Can you work these out from the model? Positions are in its coordinate system, mm. A direction names the side the tool comes from. Give positions to 0.01 mm unless a question says otherwise; leave off trailing zeros. Loops run counter-clockwise (first coordinate to the right, second up) from the corner with the lowest first, then second, coordinate; pieces in that order, holes last. Notation, with made-up numbers: (67, 69) -> (115, 69) arc R10 ccw to (115, 75) -> close; hole circle Ø11 at (7.5, -20.75). An arc over 180 degrees is marked (long way). One line per question, with ' | ' between items.
from build123d import *

# Parameters (mm, degrees)
F0_R      = 0.6477
F0_R_2    = 0.6441405576
F1_DEPTH  = 25.4
F2_W      = 127.2426065671
F2_H      = 43.082173756
F3_DEPTH  = 25.4
F6_DEPTH  = 127.2436065671
F7_W      = 127.2426065671
F7_H      = 36.2138515522
F8_DEPTH  = 25.4
F11_DEPTH = 127.2436065671
F12_W     = 127.2426065671
F12_H     = 79.2960253082
F13_DEPTH = 2.54


# Not quite as in the source:
# - ends of sketch curves that miss each other by under 0.0002 mm in the source are joined


with BuildPart() as f1:
    # F0 (on Top) → F1 (new body)
    with BuildSketch(Plane.XY):
        Polygon((-47.2229928794, 27.8801387091), (-47.2229928794, 30.4201387091), (-44.6829928794, 30.4201387091), (2.3896338216, 30.4201387091), (2.3896338216, 33.6738515522), (2.3896338216, 36.2138515522), (-62.2987892685, 36.2138515522), (-62.2987892685, 19.4619052569), (-59.7587892685, 19.4619052569), (-47.2229928794, 19.4619052569), align=None)
        Polygon((-44.6829928794, 30.4201387091), (-47.2229928794, 30.4201387091), (-47.2229928794, 27.8801387091), (-47.2229928794, 19.4619052569), (-59.7587892685, 19.4619052569), (-62.2987892685, 19.4619052569), (-62.2987892685, 16.9219052569), (-62.2987892685, -29.6174437481), (-62.2987892685, -32.1574437481), (-59.7587892685, -32.1574437481), (-16.2234111885, -32.1574437481), (-13.6834111885, -32.1574437481), (-13.6834111885, -29.6174437481), (-13.6834111885, -19.4574437481), (9.1386072609, -19.4574437481), (9.1386072609, -40.542173756), (9.1386072609, -43.082173756), (11.6786072609, -43.082173756), (32.1430532363, -43.082173756), (34.6830532363, -43.082173756), (34.6830532363, -40.542173756), (34.6830532363, -19.4574437481), (62.4038172987, -19.4574437481), (62.4038172987, -16.9174437481), (34.6830532363, -16.9174437481), (32.1430532363, -16.9174437481), (32.1430532363, -19.4574437481), (32.1430532363, -40.542173756), (11.6786072609, -40.542173756), (11.6786072609, -19.4574437481), (11.6786072609, -16.9174437481), (9.1386072609, -16.9174437481), (-13.6834111885, -16.9174437481), (-16.2234111885, -16.9174437481), (-16.2234111885, -19.4574437481), (-16.2234111885, -29.6174437481), (-59.7587892685, -29.6174437481), (-59.7587892685, 1.3920115222), (-59.7587892685, 2.6620115222), (-59.7587892685, 16.9219052569), (-47.2229928794, 16.9219052569), (-45.9529928794, 16.9219052569), (-44.6829928794, 16.9219052569), (-44.6829928794, 19.4619052569), (-44.6829928794, 27.8801387091), (2.3896338216, 27.8801387091), (4.9296338216, 27.8801387091), (4.9296338216, 30.4201387091), (4.9296338216, 33.6738515522), (11.6786072609, 33.6738515522), (11.6786072609, 30.4201387091), (11.6786072609, 27.8801387091), (14.2186072609, 27.8801387091), (62.4038172987, 27.8801387091), (62.4038172987, 30.4201387091), (14.2186072609, 30.4201387091), (14.2186072609, 33.6738515522), (14.2186072609, 36.2138515522), (11.6786072609, 36.2138515522), (4.9296338216, 36.2138515522), (2.3896338216, 36.2138515522), (2.3896338216, 33.6738515522), (2.3896338216, 30.4201387091), align=None)
        with Locations((-61.0287892685, -30.8874437481)):
            Circle(F0_R, mode=Mode.SUBTRACT)
        with Locations((-14.9534111885, -30.8874437481)):
            Circle(F0_R, mode=Mode.SUBTRACT)
        with Locations((-14.9534111885, -18.1874437481)):
            Circle(F0_R, mode=Mode.SUBTRACT)
        with Locations((10.4086072609, -41.812173756)):
            Circle(F0_R, mode=Mode.SUBTRACT)
        with Locations((33.4130532363, -41.812173756)):
            Circle(F0_R, mode=Mode.SUBTRACT)
        with Locations((10.4086072609, -18.1874437481)):
            Circle(F0_R, mode=Mode.SUBTRACT)
        with Locations((33.4130532363, -18.1874437481)):
            Circle(F0_R, mode=Mode.SUBTRACT)
        with Locations((-61.0287892685, 18.1919052569)):
            Circle(F0_R, mode=Mode.SUBTRACT)
        with Locations((-45.9529928794, 18.1919052569)):
            Circle(F0_R, mode=Mode.SUBTRACT)
        with Locations((-45.9529928794, 29.1501387091)):
            Circle(F0_R_2, mode=Mode.SUBTRACT)
        with Locations((3.6596338216, 29.1501387091)):
            Circle(F0_R, mode=Mode.SUBTRACT)
        with Locations((12.9486072609, 29.1501387091)):
            Circle(F0_R, mode=Mode.SUBTRACT)
        with Locations((3.6596338216, 34.9438515522)):
            Circle(F0_R, mode=Mode.SUBTRACT)
        with Locations((12.9486072609, 34.9438515522)):
            Circle(F0_R, mode=Mode.SUBTRACT)
        Polygon((64.9438172987, 36.2138515522), (14.2186072609, 36.2138515522), (14.2186072609, 33.6738515522), (14.2186072609, 30.4201387091), (62.4038172987, 30.4201387091), (64.9438172987, 30.4201387091), align=None)
        Polygon((-59.7587892685, -32.1574437481), (-62.2987892685, -32.1574437481), (-62.2987892685, -43.082173756), (9.1386072609, -43.082173756), (9.1386072609, -40.542173756), (9.1386072609, -19.4574437481), (-13.6834111885, -19.4574437481), (-13.6834111885, -29.6174437481), (-13.6834111885, -32.1574437481), (-16.2234111885, -32.1574437481), align=None)
        Polygon((64.9438172987, 27.8801387091), (64.9438172987, 30.4201387091), (62.4038172987, 30.4201387091), (62.4038172987, 27.8801387091), (62.4038172987, 2.6620115222), (62.4038172987, 1.3920115222), (62.4038172987, -16.9174437481), (62.4038172987, -19.4574437481), (64.9438172987, -19.4574437481), (64.9438172987, -16.9174437481), align=None)
        with Locations((63.6738172987, -18.1874437481)):
            Circle(F0_R, mode=Mode.SUBTRACT)
        with Locations((63.6738172987, 29.1501387091)):
            Circle(F0_R, mode=Mode.SUBTRACT)
        Polygon((64.9438172987, -43.082173756), (64.9438172987, -19.4574437481), (62.4038172987, -19.4574437481), (34.6830532363, -19.4574437481), (34.6830532363, -40.542173756), (34.6830532363, -43.082173756), align=None)
    extrude(amount=F1_DEPTH)

    # F2 (on face) → F3 (join)
    with BuildSketch(Plane.XY.offset(25.4)):
        with Locations((1.3225140151, -21.541086878)):
            Rectangle(F2_W, F2_H)
    extrude(amount=F3_DEPTH)

    # F5 (on face) → F6 (cut, through all)
    with BuildSketch(Plane.YZ.offset(64.9438172987)):
        Polygon((-43.082173756, 50.8), (-43.082173756, 25.4001487046), (0, 50.7993288338), (0, 50.8), align=None)
    extrude(amount=-F6_DEPTH, mode=Mode.SUBTRACT)

    # F7 (on face) → F8 (join)
    with BuildSketch(Plane.XY.offset(25.4)):
        with Locations((1.3225140151, 18.1069257761)):
            Rectangle(F7_W, F7_H)
    extrude(amount=F8_DEPTH)

    # F9 (on face) → F11 (cut, through all)
    with BuildSketch(Plane(origin=(-62.2987892685, 0, 0), x_dir=(0, -1, 0), z_dir=(-1, 0, 0))):
        Polygon((-36.2138515522, 25.4), (0, 50.7996644169), (0, 50.8), (-36.2138515522, 50.8), align=None)
    extrude(amount=-F11_DEPTH, mode=Mode.SUBTRACT)

    # F12 (on face) → F13 (join)
    with BuildSketch(Plane(origin=(0, 0, 0), x_dir=(1, 0, 0), z_dir=(0, 0, -1))):
        with Locations((1.3225140151, 3.4341611019)):
            Rectangle(F12_W, F12_H)
    extrude(amount=F13_DEPTH)


solid = f1.part
Q1. If we mould it in two halves opening along Z, with no side actions, what happens to faces 1 (the face through (0.43, 18.36, 37.92)), 2 (the face through (0, -4, 0)), 3 (the face through (-62.299, -3, 19))? For each: pulls with the +Z half, pulls with the -Z half, needs draft (parallel to the pull), parting line crosses it, or undercut.
Entries:
face 1: pulls with the +Z half | face 2: undercut | face 3: needs draft
Q2. On a 3-axis mill with a long thin cutter (end or side, diameter ignored), from which of +Z, -Z, +X, -X, +Y, -Y can I reach the whole of each face in a straight line? I mean faces 4 (the face through (8, 33.674, 13)), 5 (the face through (2.213, -21.843, 37.922)). Say none if no direction works.
Entries:
face 4: none | face 5: +Z, +X, -X, -Y
Q3. If we section it at C-C (y = -24.5): Write out the boundary of the cut face in (x, z).
Entries:
outline: (-62.3, -2.54) -> (64.94, -2.54) -> (64.94, 36.36) -> (-62.3, 36.36) -> close; hole (-59.76, 0) -> (-16.22, 0) -> (-16.22, 25.4) -> (-59.76, 25.4) -> close; hole (11.68, 0) -> (32.14, 0) -> (32.14, 25.4) -> (11.68, 25.4) -> close
Q4. If we section it at B-B (y = -4): Write out the boundary of the cut face in (x, z).
Entries:
outline: (-62.3, -2.54) -> (64.94, -2.54) -> (64.94, 48.44) -> (-62.3, 48.44) -> close; hole (-59.76, 0) -> (62.4, 0) -> (62.4, 25.4) -> (-59.76, 25.4) -> close
Q5. For pin 1 Ø1.4 at (x, y) = (-15, -31) entering from +Z; pin 2 Ø6 at (x, y) = (-21, -25) entering from +Z; pin 3 Ø10 at (x, y) = (27, 10) entering from +Z, each with a flat end and sliding along its axis, tell me the tip position at first contact or that it passes through.
Entries:
pin 1: z = 32.94 | pin 2: z = 37.83 | pin 3: z = 47.29
Q6. If I drill on probe 1 along X at (y, z) = (-19.5, 5); probe 2 along X at (y, z) = (-37.5, 3); probe 3 along X at (y, z) = (-2, 23), over which ranges is the centre line in solid material (lowest first)? Write a range as from..to.
Entries:
probe 1: -62.3..-59.76, -16.22..11.68, 32.14..64.94 | probe 2: -62.3..11.68, 32.14..64.94 | probe 3: -62.3..-59.76, 62.4..64.94
